Read the model definition and answer for the solid it produces. Units are mm, in the model's axes. A direction names the side the tool comes from. Round coordinates to 2 decimals unless told otherwise and drop trailing zeros. Order: outer loops, then holes, each group sorted by start corner. A loop starts at its lowest first (then second) coordinate and runs counter-clockwise, first axis right, second up. Notation, with made-up numbers: (64, -1.5) -> (83, -1.5) arc R27 ccw to (83, 17.5) -> close; hole circle Ø7 at (21, -24.5). An arc over 180 degrees is marked (long way). Answer as a JSON object with one key per item and string values. Group by question number.
Item 1: The mould has two halves that part along Y. Classify faces 6 (the flat face through (0, 37, 1)), 7 (the flat face through (24.5, -1, 1)), 8 (the flat face through (-15, 9.5, 8)), 9 (the flat face through (0, -37, 7)): pulls with the +Y half, pulls with the -Y half, needs draft (parallel to the pull), parting line crosses it, or undercut.
Item 2: Section C-C, the plane x = 21.3 is taken. Write down the section's boundary in (y, z), plus the area to 3 significant figures.
Item 3: Section B-B, the plane y = -14 is taken. Write down the section's boundary in (x, z), plus the area to 3 significant figures.
Item 4: Section A-A, the plane z = 13 is taken. Write down the section's boundary in (x, y).
Item 5: Section D-D, the plane y = -33.95 is taken. Write down the section's boundary in (x, z), plus the area to 3 significant figures.
Item 6: Consider probe 1 along X at (y, z) = (-2, 0.5); probe 2 along Z at (x, y) = (22, -13.5); probe 3 along X at (y, z) = (-10, 13.5). Determine where each line is inside the solid, lowest interval first. Write a range as from..to.
Item 7: Given P1, Ø1, axis at y = -1, z = 6, coming from the +X side; P2, Ø0.6, axis at x = -20.5, z = 7, coming from the +Y side; P3, Ø2, axis at x = -21, y = -34.5, coming from the +Z side; P4, Ø2.5, axis at x = -21.3, y = 33.95, coming from the -Z side, each flat-ended and moving along its own axis, determine where each tip first touches the part or whether it passes through.
Item 8: For faces 1 (the flat face through (20, 35, 6.6)), 2 (the flat face through (-23, 34, 6.6)), 3 (the flat face through (-25, 10, 3)), 4 (the flat face through (-27, -5, 1.6)), 5 (the flat face through (2, 8, 8)), determine the directions among +Z, -Z, +X, -X, +Y, -Y from which every point of the face is accessible in a straight line to the end or side of a thin tool.
from build123d import *

# Parameters (mm, degrees)
EXTRUDE_1_DEPTH     = 1.6
SKETCH_2_R          = 1.5
CUT_EXTRUDE_1_DEPTH = 45.405067278
EXTRUDE_START       = 5
SKETCH_5_R          = 2.2
SKETCH_5_R_2        = 1.5
EXTRUDE_2_DEPTH     = 5
SKETCH_6_W          = 30
SKETCH_6_H          = 45
EXTRUDE_3_DEPTH     = 13
SKETCH_7_W          = 5
SKETCH_7_H          = 30
EXTRUDE_4_DEPTH     = 3


with BuildPart() as part:
    # 草图1 → 凸台-拉伸1 (new body)
    with BuildSketch(Plane.XY):
        with BuildLine():
            Line((-23.5, -37), (23.5, -37))
            ThreePointArc((23.5, -37), (24.207106781, -36.707106781), (24.5, -36))
            Line((24.5, -36), (24.5, 36))
            ThreePointArc((24.5, 36), (24.207106781, 36.707106781), (23.5, 37))
            Line((23.5, 37), (-23.5, 37))
            ThreePointArc((-23.5, 37), (-24.207106781, 36.707106781), (-24.5, 36))
            Line((-24.5, 36), (-24.5, -36))
            ThreePointArc((-24.5, -36), (-24.207106781, -36.707106781), (-23.5, -37))
        make_face()
    extrude(amount=EXTRUDE_1_DEPTH)

    # 草图2 → 切除-拉伸1 (cut, through all)
    with BuildSketch(Plane.XY.offset(1.6)):
        with Locations((21.3, 33.95)):
            Circle(SKETCH_2_R)
        with Locations((-21.3, 33.95)):
            Circle(SKETCH_2_R)
        with Locations((-21.3, -33.95)):
            Circle(SKETCH_2_R)
        with Locations((21.3, -33.95)):
            Circle(SKETCH_2_R)
    extrude(amount=-CUT_EXTRUDE_1_DEPTH, mode=Mode.SUBTRACT)

    # 草图5 → 凸台-拉伸2 (add)
    # profile 1 of 4: a face of its own
    with BuildSketch(Plane.XY.offset(1.6).offset(EXTRUDE_START)):
        with Locations(Location((-21.3, 33.95, 0), (0, 0, 180))):
            Circle(SKETCH_5_R)
        with Locations((-21.3, 33.95)):
            Circle(SKETCH_5_R_2, mode=Mode.SUBTRACT)
    # profile 2 of 4: a face of its own
    with BuildSketch(Plane.XY.offset(1.6).offset(EXTRUDE_START)):
        with Locations(Location((21.3, -33.95, 0), (0, 0, 180))):
            Circle(SKETCH_5_R)
        with Locations((21.3, -33.95)):
            Circle(SKETCH_5_R_2, mode=Mode.SUBTRACT)
    # profile 3 of 4: a face of its own
    with BuildSketch(Plane.XY.offset(1.6).offset(EXTRUDE_START)):
        with Locations(Location((-21.3, -33.95, 0), (0, 0, 180))):
            Circle(SKETCH_5_R)
        with Locations((-21.3, -33.95)):
            Circle(SKETCH_5_R_2, mode=Mode.SUBTRACT)
    # profile 4 of 4: a face of its own
    with BuildSketch(Plane.XY.offset(1.6).offset(EXTRUDE_START)):
        with Locations(Location((21.3, 33.95, 0), (0, 0, 180))):
            Circle(SKETCH_5_R)
        with Locations((21.3, 33.95)):
            Circle(SKETCH_5_R_2, mode=Mode.SUBTRACT)
    extrude(amount=-EXTRUDE_2_DEPTH)

    # 草图6 → 凸台-拉伸3 (add)
    with BuildSketch(Plane.XY.offset(1.6)):
        Polygon((-8.5, 9.5), (-21.5, 9.5), (-21.5, 22.5), (-19.5, 22.5), (-19.5, 32.5), (9.5, 32.5), (9.5, 20), (-8.5, 20), align=None)
        with Locations((2, -14.5)):
            Rectangle(SKETCH_6_W, SKETCH_6_H)
    extrude(amount=EXTRUDE_3_DEPTH)

    # 草图7 → 凸台-拉伸4 (add)
    with BuildSketch(Plane.XY.offset(1.6)):
        with Locations((-27, -5)):
            Rectangle(SKETCH_7_W, SKETCH_7_H)
        Polygon((-24.5, 10), (-24.5, -20), (-18.5, -20), (-18.5, 9.5), (-21.5, 9.5), (-21.5, 10), align=None)
    extrude(amount=EXTRUDE_4_DEPTH)


solid = part.part
Values found:
{
 "1": {"face 6": "pulls with the +Y half", "face 7": "needs draft", "face 8": "undercut", "face 9": "pulls with the -Y half"},
 "2": {"outline": "(-37, 0) -> (-35.45, 0) -> (-35.45, 6.6) -> (-36.15, 6.6) -> (-36.15, 1.6) -> (-37, 1.6) -> close; (-32.45, 0) -> (32.45, 0) -> (32.45, 6.6) -> (31.75, 6.6) -> (31.75, 1.6) -> (-31.75, 1.6) -> (-31.75, 6.6) -> (-32.45, 6.6) -> close; (35.45, 0) -> (37, 0) -> (37, 1.6) -> (36.15, 1.6) -> (36.15, 6.6) -> (35.45, 6.6) -> close", "area": "123 mm2"},
 "3": {"outline": "(-29.5, 1.6) -> (-24.5, 1.6) -> (-24.5, 0) -> (24.5, 0) -> (24.5, 1.6) -> (17, 1.6) -> (17, 14.6) -> (-13, 14.6) -> (-13, 1.6) -> (-18.5, 1.6) -> (-18.5, 4.6) -> (-29.5, 4.6) -> close", "area": "501 mm2"},
 "4": {"outline": "(-21.5, 9.5) -> (-8.5, 9.5) -> (-8.5, 20) -> (9.5, 20) -> (9.5, 32.5) -> (-19.5, 32.5) -> (-19.5, 22.5) -> (-21.5, 22.5) -> close; (-13, -37) -> (17, -37) -> (17, 8) -> (-13, 8) -> close"},
 "5": {"outline": "(-24.5, 0) -> (-22.8, 0) -> (-22.8, 6.6) -> (-23.5, 6.6) -> (-23.5, 1.6) -> (-24.5, 1.6) -> close; (-19.8, 0) -> (19.8, 0) -> (19.8, 6.6) -> (19.1, 6.6) -> (19.1, 1.6) -> (17, 1.6) -> (17, 14.6) -> (-13, 14.6) -> (-13, 1.6) -> (-19.1, 1.6) -> (-19.1, 6.6) -> (-19.8, 6.6) -> close; (22.8, 0) -> (24.5, 0) -> (24.5, 1.6) -> (23.5, 1.6) -> (23.5, 6.6) -> (22.8, 6.6) -> close", "area": "473 mm2"},
 "6": {"probe 1": "-24.5..24.5", "probe 2": "0..1.6", "probe 3": "-13..17"},
 "7": {"P1": "x = 17", "P2": "y = 22.5", "P3": "z = 6.6", "P4": "through"},
 "8": {"face 1": "+Z, +X, +Y, -Y", "face 2": "+Z, -X, +Y", "face 3": "+Z, -X", "face 4": "-Z, -X, +Y, -Y", "face 5": "+Z, +X"}
}
